Here's how the part is built. I have some questions about the finished solid (model axes, mm). Face numbers are marked on the shaded views. A direction names the side the tool comes from. Give positions to 0.01 mm unless a question says otherwise; leave off trailing zeros.
Q1. If we section it at A-A (z = 0): Give the number of separate pieces and of enclosed holes in the cut face, plus the area to 3 significant figures.
Q2. I need wall thicknesses on line 1 (X direction, y = -37, z = 65); line 2 (X direction, y = -90, z = -99.5); line 3 (Y direction, x = -0.75, z = -62.5). Which ranges of each line are inside material? Lowest first, please.
Q3. Will these pins go through, and if not, where does the flat tip stop? P1, Ø25, axis at y = -7, z = -6.5, coming from the +X side; P2, Ø3, axis at y = -33.5, z = -89.5, coming from the -X side; P3, Ø5, axis at x = -0.5, y = -0.5, coming from the +Z side.
Q4. For the marked faces 1, 2, 3 and 4, which set-ups out of +Z, -Z, +X, -X, +Y, -Y let a thin tool reach every point of the face, with its end or its side?
Q5. We'd pull the mould along Z, two halves only. Please class the marked faces 5, 6 and 7: +Z half, -Z half, draft (parallel to the pull), parting line (faces both ways), or undercut.
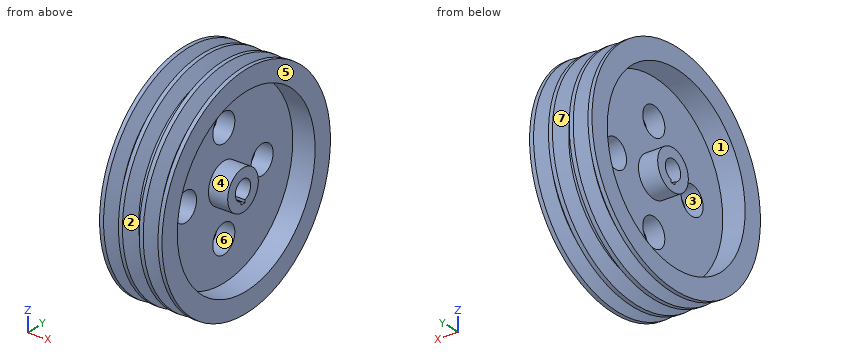
from build123d import *

# Parameters (mm, degrees)
SKETCH3_W           = 3.5
SKETCH3_H           = 6
CUT_EXTRUDE9_DEPTH  = 209.058885895
SKETCH7_R           = 18
CUT_EXTRUDE10_DEPTH = 201.779730053


with BuildPart() as part:
    # Sketch1 → Revolve5 (revolve)
    with BuildSketch(Plane.XY, mode=Mode.PRIVATE) as revolve5_sk:
        Polygon((10.452306897, 137.5), (15.452306897, 137.5), (22.003771114, 119.5), (27.448535783, 119.5), (34, 137.5), (39, 137.5), (39, 112.5), (11, 112.5), (11, 25), (35, 25), (35, 12.5), (-35, 12.5), (-35, 25), (-11, 25), (-11, 112.5), (-39, 112.5), (-39, 137.5), (-34, 137.5), (-27.448535783, 119.5), (-22.003771114, 119.5), (-15.452306897, 137.5), (-10.452306897, 137.5), (-3.900842681, 119.5), (3.900842681, 119.5), align=None)
    revolve(revolve5_sk.sketch.rotate(Axis((-35, 0, 0), (1, 0, 0)), 90), axis=Axis((-35, 0, 0), (1, 0, 0)))

    # Sketch3 → Cut-Extrude9 (cut, through all)
    with BuildSketch(Plane(origin=(35, 0, 0), x_dir=(0, 0, -1), z_dir=(1, 0, 0))):
        with Locations((13.75, 0)):
            Rectangle(SKETCH3_W, SKETCH3_H)
    extrude(amount=-CUT_EXTRUDE9_DEPTH, mode=Mode.SUBTRACT)

    # Sketch7 → Cut-Extrude10 (cut, through all)
    with BuildSketch(Plane(origin=(11, 0, 0), x_dir=(0, 0, -1), z_dir=(1, 0, 0))):
        with Locations((0, 62.5)):
            Circle(SKETCH7_R)
        with Locations((62.5, 0)):
            Circle(SKETCH7_R)
        with Locations((0, -62.5)):
            Circle(SKETCH7_R)
        with Locations((-62.5, 0)):
            Circle(SKETCH7_R)
    extrude(amount=-CUT_EXTRUDE10_DEPTH, mode=Mode.SUBTRACT)


solid = part.part
Check sheet entries:
1. separate pieces: 4
1. enclosed holes: 0
1. area: 6,540 mm2
2. line 1: x = -11 to 11
2. line 2: x = -39 to -32.79, -16.67 to -9.24, 9.24 to 16.67, 32.79 to 39
2. line 3: y = -101.85 to -18, 18 to 101.85
3. P1: stops at x = 35
3. P2: stops at x = -11
3. P3: stops at z = 119.5
4. face 1: -X
4. face 2: none
4. face 3: +X, -X
4. face 4: +X
5. face 5: draft
5. face 6: undercut
5. face 7: parting line
